```python
from build123d import *

# Parameters (mm, degrees)
F1_DEPTH = 4.572
F3_DEPTH = 12.7


with BuildPart() as f1:
    # F0 (on Top) → F1 (new body)
    with BuildSketch(Plane.XY):
        with BuildLine():
            Line((24.051455, 5.270794), (-43.004545, 5.270794))
            Line((-43.004545, 5.270794), (-43.004545, 2.095794))
            Line((-43.004545, 2.095794), (10.970455, 2.095794))
            ThreePointArc((10.970455, 2.095794), (14.145455, -1.079206), (10.970455, -4.254206))
            Line((10.970455, -4.254206), (-43.004545, -4.254206))
            Line((-43.004545, -4.254206), (-43.004545, -7.429206))
            Line((-43.004545, -7.429206), (24.051455, -7.429206))
            Line((24.051455, -7.429206), (24.051455, 5.270794))
        make_face()
    extrude(amount=F1_DEPTH)

    # F2 (on face) → F3 (join)
    with BuildSketch(Plane.XZ.offset(7.429206)):
        with BuildLine():
            Line((24.051455, 0), (12.240455, 0))
            ThreePointArc((12.240455, 0), (15.415455, -3.175), (12.240455, -6.35))
            Line((12.240455, -6.35), (-43.004545, -6.35))
            Line((-43.004545, -6.35), (-42.99381, -15.748))
            Line((-42.99381, -15.748), (24.051455, -15.748))
            Line((24.051455, -15.748), (24.051455, 0))
        make_face()
    extrude(amount=-F3_DEPTH)


with BuildPart() as f1_1:
    # F4: moved
    add(f1.part.moved(Location((43.0022, 7.4168, 15.748))))


solid = f1_1.part
```
Input: part model. Units: mm. Frame: model coordinates. A direction names the side the tool comes from. Coordinates: 2 decimals unless noted, no trailing zeros. Order: outer loops, then holes, each group sorted by start corner. A loop starts at its lowest first (then second) coordinate and runs counter-clockwise, first axis right, second up. Notation, with made-up numbers: (4.25, 44) - (34.25, 44) arc R17 cw to (34.25, 68) - close; hole circle Ø4 at (27, -32.5). An arc over 180 degrees is marked (long way). Return JSON: item names as keys, results as strings.
Q1. Access query for faces 1 (the flat face through (28, 6, 9.398)), 2 (the flat face through (41, 11, 20.32)), 3 (the flat face through (27, 9.513, 18)). Directions: +Z, -Z, +X, -X, +Y, -Y. A direction counts if a zero-diameter tool reaches every point of the face in a straight line with its end or side. Return the directions, or none.
The answers:
{"face 1": "-X, +Y, -Y", "face 2": "+Z, +X, -X, +Y, -Y", "face 3": "+Z, -X"}
Q2. Cut plane D-D (z = 13). Return loops of the section in (x, y).
The answers:
{"outline": "(58.39, -0.01) - (67.05, -0.01) - (67.05, 12.69) - (58.39, 12.69) - close"}
Q3. Cut plane A-A (x = 25). Return loops of the section in (y, z), then the cut area to 3 significant figures.
The answers:
{"outline": "(-0.01, 0) - (12.69, 0) - (12.69, 9.4) - (-0.01, 9.4) - close; (-0.01, 15.75) - (3.16, 15.75) - (3.16, 20.32) - (-0.01, 20.32) - close; (9.51, 15.75) - (12.69, 15.75) - (12.69, 20.32) - (9.51, 20.32) - close", "area": "148 mm2"}
Q4. Draft query along Y for faces 4 (the flat face through (-0.002, 2, 18)), 5 (the flat face through (27, 3.163, 18)), 6 (the cylindrical face through (57.147, 6.407, 18.002)), 7 (the flat face through (33, 12.688, 8)). Return one class per face: +Y half, -Y half, draft (parallel to the pull), parting line (faces both ways), or undercut.
The answers:
{"face 4": "draft", "face 5": "undercut", "face 6": "undercut", "face 7": "+Y half"}
Q5. Cut plane B-B (y = 2). Return loops of the section in (x, z) (3 decimals), then the cut area to 3 significant figures.
The answers:
{"outline": "(-0.002, 9.398) - (0.008, 0) - (67.054, 0) - (67.054, 20.32) - (-0.002, 20.32) - (-0.002, 15.748) - (55.243, 15.748) arc R3.175 cw to (55.243, 9.398) - close", "area": "996 mm2"}
Q6. First-contact query: pin 1 (6 mm diameter, centred on x = 16.5, z = 12.5, fed in from -Y). Flat tip, straight axial feed; report the tip coordinate or a pass-through.
The answers:
{"pin 1": "passes through"}
Q7. Cut plane C-C (x = 56). Return loops of the section in (y, z).
The answers:
{"outline": "(-0.01, 0) - (12.69, 0) - (12.69, 9.49) - (-0.01, 9.49) - close; (-0.01, 15.66) - (12.69, 15.66) - (12.69, 20.32) - (8.78, 20.32) - (8.78, 15.75) - (3.89, 15.75) - (3.89, 20.32) - (-0.01, 20.32) - close"}
Q8. Ray query, probe 1 along Z at (x, y) = (55, 1); probe 2 along Y at (x, z) = (48, 18.5); probe 3 along Z at (x, y) = (39.5, 4.25). Return the intervals inside material, ascending.
The answers:
{"probe 1": "z = 0 to 9.4, 15.75 to 20.32", "probe 2": "y = -0.01 to 3.16, 9.51 to 12.69", "probe 3": "z = 0 to 9.4"}
